Geometry: final body of the model. Coordinates: model frame, mm. Face numbers are marked on the shaded views. A direction names the side the tool comes from. Give positions to 0.01 mm unless a question says otherwise; leave off trailing zeros. Write each loop counter-clockwise with the first axis right and the second up, starting at its lowest first coordinate (ties: lowest second). Pieces come first, ordered by that corner, then holes. Notation, with made-up numbers: M 44,80.25 L 90,80.25 A37 cw 90,118.25 Z; hole C 83,25 d11. An arc over 180 degrees is marked long. One line per question, with ' | ' between items.
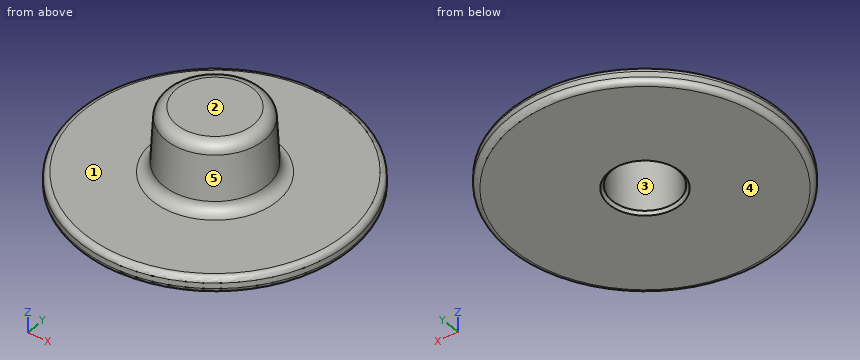
from build123d import *

# Parameters (mm, degrees)
HOLE_D           = 6
HOLE_DEPTH       = 6.5
HOLE_CSINK_D     = 6.5
HOLE_CSINK_ANGLE = 90


with BuildPart() as part:
    # Sketch → Revolution (revolve)
    with BuildSketch(Plane.XZ):
        with BuildLine():
            Line((12.5, 1), (12.5, 0.5))
            ThreePointArc((12, 0), (12.353553, 0.146447), (12.5, 0.5))
            Line((12, 0), (0, 0))
            Line((0, 7.5), (0, 0))
            Line((3.5, 7.5), (0, 7.5))
            ThreePointArc((4.49863, 6.552336), (4.188355, 7.225374), (3.5, 7.5))
            Line((4.49863, 6.552336), (4.713746, 2.447664))
            ThreePointArc((4.713746, 2.447664), (5.024021, 1.774626), (5.712376, 1.5))
            Line((5.712376, 1.5), (12, 1.5))
            ThreePointArc((12.5, 1), (12.353553, 1.353553), (12, 1.5))
        make_face()
    revolve(axis=Axis((0, 0, 0), (0, 0, 1)))

    # Hole
    with Locations(Plane(origin=(0, 0, 0), x_dir=(1, 0, 0), z_dir=(0, 0, -1))):
        with Locations((0, 0)):
            CounterSinkHole(HOLE_D / 2, HOLE_CSINK_D / 2, depth=HOLE_DEPTH, counter_sink_angle=HOLE_CSINK_ANGLE)


solid = part.part
(1) First-contact query: P1, Ø6, axis at x = 7, y = -4.5, coming from the +Z side; P2, Ø3, axis at x = 0.5, y = 1, coming from the -Z side; P3, Ø6, axis at x = 8, y = 0, coming from the +Z side; P4, Ø2, axis at x = -6.5, z = 4, coming from the -Y side. Flat tips, straight axial feed; report the tip coordinate or a pass-through.
Working result:
P1: stops at z = 1.58 | P2: stops at z = 6.5 | P3: stops at z = 1.8 | P4: passes through
(2) Material intervals for L1, parallel to Z at x = 10, y = -2.75; L2, parallel to Y at x = 0, z = 2.75; L3, parallel to Y at x = 0, z = 4.75, sorted ascending. Write a range as [from, to].
Working result:
L1: z = [0, 1.5] | L2: y = [-4.7, -3], [3, 4.7] | L3: y = [-4.59, -3], [3, 4.59]
(3) Cut plane C-C, the plane z = 6. Return loops of the section in (x, y), then the cut area to 3 significant figures.
Working result:
outline: C 0,0 d9.06; hole C 0,0 d6 | area: 36.1 mm^2
(4) Cut plane A-A, the plane y = 0. Return loops of the section in (x, z), then the cut area to 3 significant figures.
Working result:
outline: M -12.5,0.5 A0.5 ccw -12,0 L -3.25,0 L -3,0.25 L -3,6.5 L 3,6.5 L 3,0.25 L 3.25,0 L 12,0 A0.5 ccw 12.5,0.5 L 12.5,1 A0.5 ccw 12,1.5 L 5.71,1.5 A1 cw 4.71,2.45 L 4.5,6.55 A1 ccw 3.5,7.5 L -3.5,7.5 A1 ccw -4.5,6.55 L -4.71,2.45 A1 cw -5.71,1.5 L -12,1.5 A0.5 ccw -12.5,1 Z | area: 53.5 mm^2
(5) Draft query along X for the marked faces 3, 4 and 5. Return one class per face: released by +X, released by -X, zero draft, split by the parting line, or undercut.
Working result:
face 3: undercut | face 4: zero draft | face 5: split by the parting line
(6) Cut plane D-D, the plane z = 4.5. Return loops of the section in (x, y), then the cut area to 3 significant figures.
Working result:
outline: C 0,0 d9.21; hole C 0,0 d6 | area: 38.4 mm^2
(7) Set-up query: the marked faces 1 and 2. Return all of +Z, -Z, +X, -X, +Y, -Y with unobstructed straight access to the full face (end or side cutting, diameter ignored); none if empty.
Working result:
face 1: +Z | face 2: +Z, +X, -X, +Y, -Y
